Geometry check sheet. Reference: the model listing, model coordinates, mm. A direction names the side the tool comes from. Give positions to 0.01 mm unless a question says otherwise; leave off trailing zeros. Write each loop counter-clockwise with the first axis right and the second up, starting at its lowest first coordinate (ties: lowest second). Pieces come first, ordered by that corner, then holes. Notation, with made-up numbers: (37, 41) -> (79, 41) arc R37 ccw to (79, 79) -> close; hole circle Ø10 at (12, 24.5). An arc over 180 degrees is marked (long way). Write item = value, one per line. Start each with the question number.
1. Thickness scan on line 1 along X through (y, z) = (1.6, -0.45); line 2 along Y through (x, z) = (8.25, 0.5); line 3 along X through (y, z) = (1.1, 0.4). Record the ranges inside material, lowest first.
2. Set-up check for faces 1 (the cylindrical face through (7, 0, 1)), 2 (the flat face through (0, 0, 1)), 3 (the flat face through (0.5, 0, -0.75)): record each of +Z, -Z, +X, -X, +Y, -Y from which the full face is reachable in a straight line by a thin tool's end or side.
3. Depth check by flat-ended pin: P1, Ø1.5, axis at x = 9.5, y = 0.5, coming from the +Z side; P2, Ø1.1, axis at y = 0, z = -1, coming from the +X side. Enter the tip coordinate at first touch or a pass-through.
4. Cross-section at A-A, the plane x = 10. Record the cut outline in (y, z), plus the area to 3 significant figures.
```python
from build123d import *

# Parameters (mm, degrees)
FILLET_1_R          = 0.5
CUT_EXTRUDE_2_DEPTH = 1
CHAMFER_3_SIZE      = 0.25


with BuildPart() as part:
    # Эскиз2 → Повернуть1 (revolve)
    with BuildSketch(Plane.XY):
        Polygon((0, 0), (0, -1.9), (2, -1.9), (2, -1), (12, -1), (12, 0), align=None)
    revolve(axis=Axis((0, 0, 0), (1, 0, 0)))

    # Скругление1
    fillet_1_edges = [part.edges().sort_by_distance(p)[0] for p in [
        (2, 1, 0),
    ]]
    fillet(fillet_1_edges, radius=FILLET_1_R)

    # Эскиз3 → Вырез-Вытянуть2 (cut)
    with BuildSketch(Plane.ZY):
        Polygon((0, 0.866025404), (-0.75, 0.433012702), (-0.75, -0.433012702), (0, -0.866025404), (0.75, -0.433012702), (0.75, 0.433012702), align=None)
    extrude(amount=-CUT_EXTRUDE_2_DEPTH, mode=Mode.SUBTRACT)

    # Эскиз5 → Вырез-Повернуть1 (revolve, cut)
    with BuildSketch(Plane.XY):
        Polygon((1, -0.866025404), (1, 0), (1.5, 0), align=None)
    revolve(axis=Axis((1, 0, 0), (1, 0, 0)), mode=Mode.SUBTRACT)

    # Фаска3
    chamfer_3_edges = [part.edges().sort_by_distance(p)[0] for p in [
        (12, 1, 0),
    ]]
    chamfer(chamfer_3_edges, length=CHAMFER_3_SIZE)


solid = part.part
```
Answers:
q1.line_1 = 0 to 2
q1.line_2 = -0.87 to 0.87
q1.line_3 = 0 to 2.12
q2.face_1 = +X
q2.face_2 = +Z, -Z, -X, +Y, -Y
q2.face_3 = -X
q3.P1 = 1
q3.P2 = 12
q4.outline = circle Ø2 at (0, 0)
q4.area = 3.14 mm^2
